Here's the drawing with two shaded views (mm, measured from the low corner). I have some questions. Give positions to 0.01 mm unless a question says otherwise; leave off trailing zeros. Order: outer loops, then holes, each group sorted by start corner. A loop starts at its lowest first (then second) coordinate and runs counter-clockwise, first axis right, second up. Notation, with made-up numbers: M -23.75,-7.5 L 2.25,-7.5 A26 ccw 2.25,17.5 Z; hole C 27,77.25 d10. An arc over 180 degrees is marked long. Write each question's results on one line, items separated by ' | '.
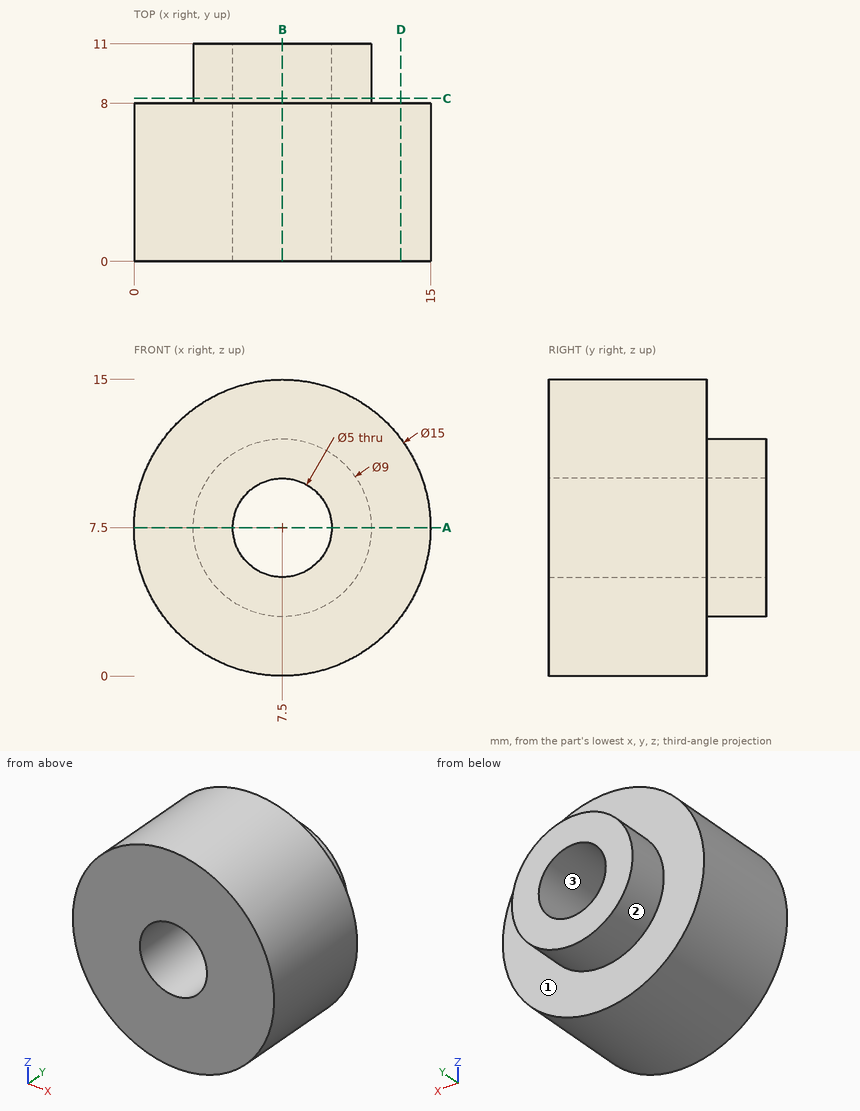
(1) Imagine slicing it at D-D, the plane x = 13.5. Write out the boundary of the cut face in (y, z).
Data:
outline: M 0,3 L 8,3 L 8,12 L 0,12 Z
(2) Imagine slicing it at A-A, the plane z = 7.5. Write out the boundary of the cut face in (x, y).
Data:
outline: M 0,0 L 5,0 L 5,11 L 3,11 L 3,8 L 0,8 Z; M 10,0 L 15,0 L 15,8 L 12,8 L 12,11 L 10,11 Z
(3) I need wall thicknesses on L1, parallel to X at y = 4, z = 7.5; L2, parallel to Y at x = 8.25, z = 1.25; L3, parallel to X at y = 8.75, z = 7.5. Which ranges of each line are inside material? Lowest first, please. Write a range as from..to.
Data:
L1: x = 0..5, 10..15 | L2: y = 0..8 | L3: x = 3..5, 10..12
(4) We'd pull the mould along Z, two halves only. Please class the marked faces 1, 2 and 3: +Z half, -Z half, draft (parallel to the pull), parting line (faces both ways), or undercut.
Data:
face 1: draft | face 2: parting line | face 3: undercut
(5) Imagine slicing it at B-B, the plane x = 7.5. Write out the boundary of the cut face in (y, z), plus the area to 3 significant figures.
Data:
outline: M 0,0 L 8,0 L 8,3 L 11,3 L 11,5 L 0,5 Z; M 0,10 L 11,10 L 11,12 L 8,12 L 8,15 L 0,15 Z | area: 92.0 mm2
(6) Will these pins go through, and if not, where does the flat tip stop? P1, Ø6.5, axis at x = 7.5, z = 7.5, coming from the +Y side; P2, Ø2, axis at x = 9, y = 5.5, coming from the -Z side; P3, Ø1.5, axis at x = 2, z = 10, coming from the +Y side; P4, Ø1, axis at x = 4, y = 8, coming from the -Z side.
Data:
P1: stops at y = 11 | P2: stops at z = 0.02 | P3: stops at y = 8 | P4: stops at z = 0.63
(7) Imagine slicing it at C-C, the plane y = 8.25. Write out the boundary of the cut face in (x, z), plus the area to 3 significant figures.
Data:
outline: C 7.5,7.5 d9; hole C 7.5,7.5 d5 | area: 44.0 mm2
